The model under review builds one solid part; all positions refer to its coordinate system, in mm. Round coordinates to 2 decimals unless told otherwise and drop trailing zeros. Write each loop counter-clockwise with the first axis right and the second up, starting at its lowest first coordinate (ties: lowest second). Pieces come first, ordered by that corner, then holes. Notation, with made-up numbers: (-35.5, 56.25) -> (0.5, 56.25) arc R21 cw to (0.5, 66.25) -> close; hole circle Ø6 at (75.25, -13). An arc over 180 degrees is marked (long way). Return JSON: item names as keys, results as strings. Group by question number.
1. Clearance check with flat-ended pins moving along their axes: P1, Ø12, axis at y = 310.5, z = -18.5, coming from the -X side; P2, Ø6, axis at x = -10, y = 481.5, coming from the +Z side; P3, Ø5, axis at x = -1, y = 499.5, coming from the +Z side. State where each tip first meets the part, or that it passes through.
2. For line 1 along Y through (x, z) = (0, 25) (3 decimals); line 2 along X through (y, z) = (500, 23) (3 decimals); line 3 along X through (y, z) = (500, 25) (3 decimals), list the stretches that pass through material, from the lowest coordinate up. Write a range as from..to.
3. Take a section at A-A, the plane y = 456. Write out the cut boundary in (x, z), then the cut area to 3 significant figures.
4. Take a section at B-B, the plane x = -18. Write out the cut boundary in (y, z), then the cut area to 3 significant figures.
from build123d import *

# Parameters (mm, degrees)
F0_W     = 45.9264908458
F0_H     = 35.4225555062
F2_DEPTH = 1000
F4_DEPTH = 1000
F5_D     = 6.35
F5_DEPTH = 11.2897222469


with BuildPart() as f2:
    # F0 (on Front) → F2 (new body)
    with BuildSketch(Plane.XZ):
        Rectangle(F0_W, F0_H)
    extrude(amount=-F2_DEPTH)

    # F0 (on Front) → F4 (join)
    with BuildSketch(Plane.XZ):
        with BuildLine():
            ThreePointArc((22.9632454229, -17.7112777531), (27.4493544302, -9.3559040914), (29, 0))
            ThreePointArc((29, 0), (27.4493544302, 9.3559040914), (22.9632454229, 17.7112777531))
            Line((22.9632454229, 17.7112777531), (22.9632454229, -17.7112777531))
        make_face()
        with BuildLine():
            Line((-22.9632454229, 17.7112777531), (22.9632454229, 17.7112777531))
            ThreePointArc((22.9632454229, 17.7112777531), (0, 29), (-22.9632454229, 17.7112777531))
        make_face()
        Rectangle(F0_W, F0_H)
        with BuildLine():
            ThreePointArc((-22.9632454229, -17.7112777531), (0, -29), (22.9632454229, -17.7112777531))
            Line((22.9632454229, -17.7112777531), (-22.9632454229, -17.7112777531))
        make_face()
        with BuildLine():
            Line((-22.9632454229, -17.7112777531), (-22.9632454229, 17.7112777531))
            ThreePointArc((-22.9632454229, 17.7112777531), (-29, 0), (-22.9632454229, -17.7112777531))
        make_face()
    extrude(amount=-F4_DEPTH)

    # F5 (through all, one way)
    with BuildSketch(Plane(origin=(0, 0, 17.7112777531), x_dir=(1, 0, 0), z_dir=(0, 0, -1))):
        with Locations((0, -500)):
            Circle(F5_D / 2)
    extrude(amount=-F5_DEPTH, mode=Mode.SUBTRACT)


solid = f2.part
Output:
{
 "1": {"P1": "stops at x = -26.17", "P2": "stops at z = 28.14", "P3": "stops at z = 28.98"},
 "2": {"line 1": "y = 0..496.825, 503.175..1000", "line 2": "x = -17.664..-3.175, 3.175..17.664", "line 3": "x = -14.697..-3.175, 3.175..14.697"},
 "3": {"outline": "circle Ø58 at (0, 0)", "area": "2,640 mm^2"},
 "4": {"outline": "(0, -22.74) -> (1000, -22.74) -> (1000, 22.74) -> (0, 22.74) -> close", "area": "45,500 mm^2"}
}
